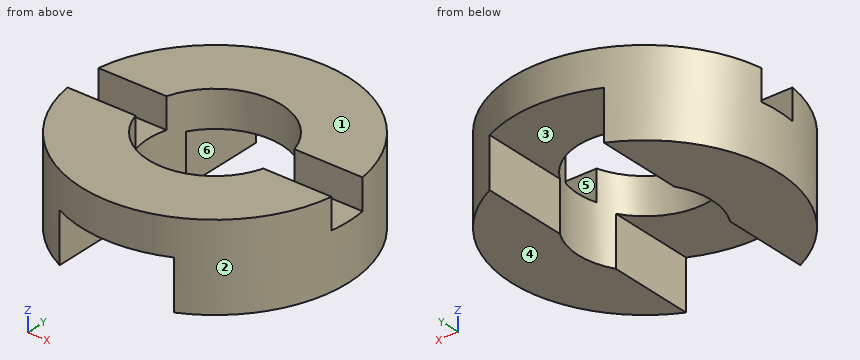
```python
from build123d import *

# Parameters (mm, degrees)
SKETCH_1_R               = 7
SKETCH_1_R_2             = 3.5
EXTRUDE_1_DEPTH          = 4.5
SKETCH_2_W               = 6
SKETCH_2_H               = 2.6
CUT_EXTRUDE_1_DEPTH      = 8
CUT_EXTRUDE_1_DEPTH_BACK = 8
SKETCH_3_W               = 1.6
SKETCH_3_H               = 2
CUT_EXTRUDE_2_DEPTH      = 8
CUT_EXTRUDE_2_DEPTH_BACK = 8


with BuildPart() as part:
    # Эскиз1 → Бобышка-Вытянуть1 (new body)
    with BuildSketch(Plane.XY):
        Circle(SKETCH_1_R)
        Circle(SKETCH_1_R_2, mode=Mode.SUBTRACT)
    extrude(amount=EXTRUDE_1_DEPTH)

    # Эскиз2 → Вырез-Вытянуть1 (cut, two sides)
    with BuildSketch(Plane(origin=(0, 0, 0), x_dir=(1, 0, 0), z_dir=(0, 1, 0))) as cut_extrude_1_sk:
        with Locations((0, -1.3)):
            Rectangle(SKETCH_2_W, SKETCH_2_H)
    extrude(amount=CUT_EXTRUDE_1_DEPTH, mode=Mode.SUBTRACT)
    extrude(cut_extrude_1_sk.sketch, amount=-CUT_EXTRUDE_1_DEPTH_BACK, mode=Mode.SUBTRACT)

    # Эскиз3 → Вырез-Вытянуть2 (cut, two sides)
    with BuildSketch(Plane(origin=(0, 0, 0), x_dir=(0, 0, -1), z_dir=(1, 0, 0))) as cut_extrude_2_sk:
        with Locations((-3.7, 0)):
            Rectangle(SKETCH_3_W, SKETCH_3_H)
    extrude(amount=CUT_EXTRUDE_2_DEPTH, mode=Mode.SUBTRACT)
    extrude(cut_extrude_2_sk.sketch, amount=-CUT_EXTRUDE_2_DEPTH_BACK, mode=Mode.SUBTRACT)


solid = part.part
```
Check sheet for the modelled part. Datum: model origin and axes. Units: mm. Face numbers are marked on the shaded views. A direction names the side the tool comes from. Round coordinates to 2 decimals unless told otherwise and drop trailing zeros. Loops run counter-clockwise (first coordinate to the right, second up) from the corner with the lowest first, then second, coordinate; pieces in that order, holes last. Notation, with made-up numbers: (56, 51.5) - (93, 51.5) arc R26 cw to (93, 80.5) - close; hole circle Ø3 at (13.25, 77.5). An arc over 180 degrees is marked (long way). Write item = value, one per line. Start each with the question number.
Q1. Thickness scan on L1, parallel to X at y = 0, z = 1.9; L2, parallel to X at y = 3, z = 3.8. Record the ranges inside material, lowest first.
Q2. Release check for a two-part mould opening along X. For the marked faces 1, 2 and 3 record: pulls with the +X half, pulls with the -X half, needs draft (parallel to the pull), parting line crosses it, or undercut.
Q3. Access from +Z, -Z, +X, -X, +Y, -Y to the whole of each face (thin tool, end or side, straight path). Record for the marked faces 4, 5 and 6.
Q4. Section check C-C (z = 0.4). Record the boundary of the cut face in (x, y).
Q5. Section check B-B (y = -3). Record the boundary of the cut face in (x, z).
Q6. Depth check by flat-ended pin: P1, Ø0.8, axis at y = -4, z = 1, coming from the +X side; P2, Ø1.3, axis at x = 6, z = 3.5, coming from the +Y side; P3, Ø0.8, axis at x = 4.5, z = 4, coming from the -Y side. Enter the tip coordinate at first touch or a pass-through.
Q7. Section check D-D (y = 5.25). Record the boundary of the cut face in (x, z).
Q8. Section check A-A (x = -1). Record the boundary of the cut face in (y, z).
Derived:
q1.L1 = -7 to -3.5, 3.5 to 7
q1.L2 = -6.32 to -1.8, 1.8 to 6.32
q2.face_1 = needs draft
q2.face_2 = parting line crosses it
q2.face_3 = undercut
q3.face_4 = -Z, +X, -X, +Y, -Y
q3.face_5 = +Z, +X, -X
q3.face_6 = -Z, +Y, -Y
q4.outline = (-3, -6.32) - (-3, -1.8) arc R3.5 cw to (-3, 1.8) - (-3, 6.32) arc R7 ccw to start; (3, -6.32) arc R7 ccw to (3, 6.32) - (3, 1.8) arc R3.5 cw to (3, -1.8) - close
q5.outline = (-6.32, 0) - (-3, 0) - (-3, 2.6) - (-1.8, 2.6) - (-1.8, 4.5) - (-6.32, 4.5) - close; (1.8, 2.6) - (3, 2.6) - (3, 0) - (6.32, 0) - (6.32, 4.5) - (1.8, 4.5) - close
q6.P1 = 6
q6.P2 = 4.51
q6.P3 = -5.67
q7.outline = (-4.63, 0) - (-3, 0) - (-3, 2.6) - (3, 2.6) - (3, 0) - (4.63, 0) - (4.63, 4.5) - (-4.63, 4.5) - close
q8.outline = (-6.93, 2.6) - (-3.35, 2.6) - (-3.35, 4.5) - (-6.93, 4.5) - close; (3.35, 2.6) - (6.93, 2.6) - (6.93, 4.5) - (3.35, 4.5) - close
